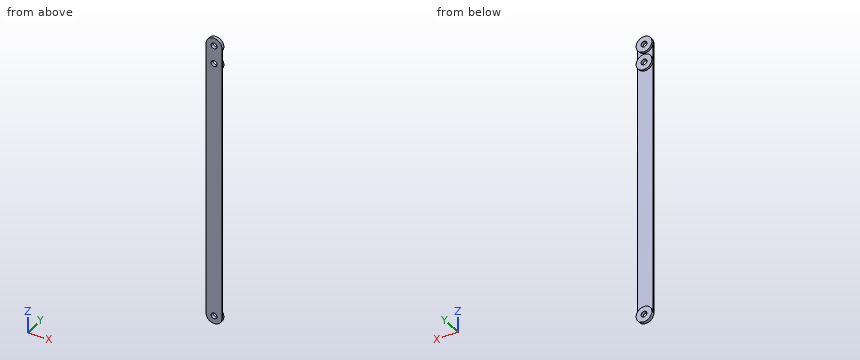
Autodesk Inventor part; units mm, degrees
ref_plane "YZ Plane" through (0, 0, 0) normal (1, 0, 0) x (0, 1, 0)
ref_plane "XZ Plane" through (0, 0, 0) normal (0, 1, 0) x (-1, 0, 0)
ref_plane "XY Plane" through (0, 0, 0) normal (0, 0, 1) x (1, 0, 0)
sketch "Sketch1" plane through (0, 0, 0) normal (0, 1, 0) x (-1, 0, 0)
  circle A0 centre (0, 0) radius 7.5
  circle A1 centre (0, 0) radius 2.75
  line L0 (-7.5, -247.97) -> (-7.5, 0)
  line L1 (7.5, 0) -> (7.5, -247.97)
  arc A2 (7.5, 0) -> (-7.5, 0) centre (0, 0) ccw
  line L2 (0, -255.47) -> (0, -240.47)
  circle A3 centre (0, -247.97) radius 2.75
  circle A4 centre (0, -247.97) radius 7.5
  line L3 (-7.5, 7.5) -> (-7.5, 10)
  line L4 (7.5, 10) -> (7.5, 7.5)
  line L5 (-7.5, 10) -> (-7.5, 17.5)
  line L6 (7.5, 17.5) -> (7.5, 10)
  circle A5 centre (0, 17.5) radius 7.5
  circle A6 centre (0, 17.5) radius 2.75
  line L7 (7.5, 7.5) -> (7.5, 0)
  line L8 (-7.5, 7.5) -> (-7.5, 0)
  line L9 (7.5, 0) -> (7.5, -247.97)
  line L10 (7.5, -123.985) -> (-7.5, -123.985)
  line L11 (-7.5, -255.47) -> (-7.5, -257.97)
  line L12 (7.5, -257.97) -> (7.5, -255.47)
  line L13 (-7.5, -257.97) -> (-7.5, -265.47)
  line L14 (7.5, -265.47) -> (7.5, -257.97)
  circle A7 centre (0, -265.47) radius 7.5
  circle A8 centre (0, -265.47) radius 2.75
  line L15 (7.5, -255.47) -> (7.5, -247.97)
  line L16 (-7.5, -255.47) -> (-7.5, -247.97)
  point P0 (7.5, 0)
  point P1 (-7.5, 0)
  point P2 (0, 7.5)
  point P3 (7.5, 0)
  dimension "d0" = 15
  dimension "d1" = 5.5
  dimension "d7" = 15
  dimension "d12" = 15
  dimension "d13" = 5.5
  dimension "d17" = 262.97
  dimension "d18" = 15
  dimension "d19" = 2.5
  dimension "d22" = 15
  dimension "d23" = 5.5
extrude "Extrusion2" add sketch "Sketch1" along normal blind 3 contours A0 | A4 L2 A3 | A4 L2 A3 | A5
extrude "Extrusion3" add sketch "Sketch1" along normal blind 1 contours L1 L10 L0 A0 | A0 L8 L3 L5 A5 L6 L4 L7 | L1 A4 L0 L10 | A5
properties part number "közepső szalag 1"
Input: part model. Units: mm. Frame: model coordinates. Give positions to 0.01 mm unless a question says otherwise; leave off trailing zeros. Order: outer loops, then holes, each group sorted by start corner. A loop starts at its lowest first (then second) coordinate and runs counter-clockwise, first axis right, second up. Notation, with made-up numbers: (-16.5, 38) -> (1.5, 38) arc R23 ccw to (1.5, 71) -> close; hole circle Ø9 at (4, -17). An arc over 180 degrees is marked (long way). Use one line per item in the form item = value.
1) First-contact query: pin 1 Ø5 at (x, z) = (0, 0) entering from +Y; pin 2 Ø1 at (x, y) = (2.5, 1.5) entering from -Z. Flat tips, straight axial feed; report the tip coordinate or a pass-through.
Response values:
pin_1 = through
pin_2 = -255.2
2) Section A-A, the plane x = 0. Return loops of the section in (y, z).
Response values:
outline = (0, -255.47) -> (3, -255.47) -> (3, -250.72) -> (0, -250.72) -> close; (0, -245.22) -> (3, -245.22) -> (3, -240.47) -> (1, -240.47) -> (1, -7.5) -> (3, -7.5) -> (3, -2.75) -> (0, -2.75) -> close; (0, 2.75) -> (3, 2.75) -> (3, 7.5) -> (1, 7.5) -> (1, 10) -> (3, 10) -> (3, 14.75) -> (0, 14.75) -> close; (0, 20.25) -> (3, 20.25) -> (3, 25) -> (0, 25) -> close
3) Section B-B, the plane y = 0.55. Return loops of the section in (x, z).
Response values:
outline = (-7.5, -247.97) arc R7.5 ccw to (7.5, -247.97) -> (7.5, 17.5) arc R7.5 ccw to (-7.5, 17.5) -> close; hole circle Ø5.5 at (0, -247.97); hole circle Ø5.5 at (0, 0); hole circle Ø5.5 at (0, 17.5)
4) Section C-C, the plane z = -150. Return loops of the section in (x, y).
Response values:
outline = (-7.5, 0) -> (7.5, 0) -> (7.5, 1) -> (-7.5, 1) -> close
5) Line query: probe 1 along Z at (x, y) = (0.25, 2.5); probe 2 along Z at (x, y) = (0, 0.7); probe 3 along Y at (x, z) = (-1.75, -138). Output: solid intervals per line, ascending.
Response values:
probe_1 = -255.47 to -250.71, -245.23 to -240.47, -7.5 to -2.74, 2.74 to 7.5, 10 to 14.76, 20.24 to 25
probe_2 = -255.47 to -250.72, -245.22 to -2.75, 2.75 to 14.75, 20.25 to 25
probe_3 = 0 to 1
